Autodesk Inventor part; units mm, degrees
ref_plane "YZ Plane" through (0, 0, 0) normal (1, 0, 0) x (0, 1, 0)
ref_plane "XZ Plane" through (0, 0, 0) normal (0, 1, 0) x (-1, 0, 0)
ref_plane "XY Plane" through (0, 0, 0) normal (0, 0, 1) x (1, 0, 0)
sketch "Sketch1" plane through (0, 0, 0) normal (1, 0, 0) x (0, 1, 0)
  line L0 (40, 0) -> (40, 3)
  line L1 (40, 3) -> (10, 3)
  line L2 (10, 3) -> (10, 6)
  arc A0 (10, 6) -> (2.1459, 3) centre (5.5, 6) ccw
  line L3 (0, 0) -> (0, 3)
  line L4 (0, 3) -> (2.1459, 3)
  line L5 (40, 0) -> (0, 0)
  circle A1 centre (5.5, 6) radius 1.5
  dimension "d7" = 3
extrude "Extrusion1" add sketch "Sketch1" along normal blind 20
sketch "Sketch2" plane through (0, 0, 0) normal (0, -1, 0) x (1, 0, 0)
  line L0 (0, 0) -> (20, 0)
  line L1 (18.5, 0) -> (16.5, 0)
  line L2 (15, 1.5) -> (15, 1.5)
  line L3 (0, 3) -> (20, 3)
  line L4 (16.5, 3) -> (18.5, 3)
  line L5 (20, 1.5) -> (20, 1.5)
  arc A0 (20, 1.5) -> (18.5, 3) centre (18.5, 1.5) ccw
  arc A1 (18.5, 0) -> (20, 1.5) centre (18.5, 1.5) ccw
  arc A2 (16.5, 3) -> (15, 1.5) centre (16.5, 1.5) ccw
  arc A3 (15, 1.5) -> (16.5, 0) centre (16.5, 1.5) ccw
  line L6 (0, 6) -> (0, 3)
  line L7 (1.5, 3) -> (3.5, 3)
  line L8 (5, 1.5) -> (5, 1.5)
  line L9 (3.5, 0) -> (1.5, 0)
  line L10 (0, 0) -> (0, 3)
  line L11 (0, 1.5) -> (0, 1.5)
  arc A4 (5, 1.5) -> (3.5, 3) centre (3.5, 1.5) ccw
  arc A5 (3.5, 0) -> (5, 1.5) centre (3.5, 1.5) ccw
  arc A6 (1.5, 3) -> (0, 1.5) centre (1.5, 1.5) ccw
  arc A7 (0, 1.5) -> (1.5, 0) centre (1.5, 1.5) ccw
  point P0 (15, 0)
  point P1 (15, 3)
  point P2 (5, 3)
  point P3 (5, 0)
  dimension "d10" = 5
  dimension "d11" = 3
  dimension "d12" = 5
  dimension "d13" = 3
  dimension "d14" = 1.5
  dimension "d15" = 5
  dimension "d16" = 3
  dimension "d17" = 5
  dimension "d18" = 3
  dimension "d19" = 1.5
extrude "Extrusion2" add sketch "Sketch2" along normal blind 19 contours A7 A6 L3 A4 A5 L0 | A3 A2 L3 A0 A1 L0
ref_plane "Work Plane1" through (18.5, -19, 3) normal (0, -1, 0) x (1, 0, 0)
sketch "Sketch4" plane through (20, 0, 0) normal (1, 0, 0) x (0, 0, -1)
  line L0 (-3, -19) -> (0, -19)
  line L1 (0, -19) -> (0, -29)
  line L2 (0, -29) -> (-6, -29)
  arc A0 (-3, -21.1459) -> (-6, -29) centre (-6, -24.5) ccw
  line L3 (-3, -19) -> (-3, -21.1459)
  circle A1 centre (-6, -24.5) radius 1.5
  point P0 (0, 0)
  dimension "d31" = 3
extrude "Extrusion3" add sketch "Sketch4" against normal blind 20
sketch "Sketch5" plane through (0, 40, 3) normal (0, 1, 0) x (1, 0, 0)
  line L0 (0, 3) -> (20, 3)
  line L1 (20, 3) -> (20, 15)
  line L2 (20, 15) -> (0, 15)
  line L3 (0, 0) -> (0, 3)
  line L4 (0, 15) -> (0, 3)
  line L5 (0, 3) -> (20, 3)
  circle A0 centre (17, 10) radius 1.5
  circle A1 centre (3, 10) radius 1.5
  dimension "d34" = 12
  dimension "d35" = 20
  dimension "d36" = 12
  dimension "d37" = 20
  dimension "d40" = 3
  dimension "d43" = 3
extrude "Extrusion4" add sketch "Sketch5" against normal blind 5
sketch "Sketch6" plane through (20, -29, 0) normal (0, -1, 0) x (1, 0, 0)
  line L0 (-20, 0) -> (-20, -12)
  line L1 (-20, 0) -> (-20, -12)
  line L2 (-20, -12) -> (0, -12)
  line L3 (-1.5, 0) -> (0, 0)
  line L4 (0, -12) -> (0, 0)
  line L5 (0, 0) -> (-20, 0)
  line L6 (-16.5, 0) -> (-3.5, 0)
  circle A0 centre (-17, -7) radius 1.5
  circle A1 centre (-17, -7) radius 1.5
  circle A2 centre (-3, -7) radius 1.5
  circle A3 centre (-3, -7) radius 1.5
  dimension "d46" = 12
  dimension "d47" = 20
  dimension "d48" = 12
  dimension "d49" = 20
  dimension "d50" = 3
  dimension "d51" = 3
extrude "Extrusion5" add sketch "Sketch6" against normal blind 5
Verification items for the finished model (mm, model axes). A direction names the side the tool comes from. Coordinates: 2 decimals unless noted, no trailing zeros. Order: outer loops, then holes, each group sorted by start corner. A loop starts at its lowest first (then second) coordinate and runs counter-clockwise, first axis right, second up. Notation, with made-up numbers: (71.5, 36) -> (100.5, 36) arc R19 ccw to (100.5, 56) -> close; hole circle Ø9 at (65.25, 37). An arc over 180 degrees is marked (long way). Put each result on its own line as item: value. Start each with the question number.
1) Go/stop test with flat-tipped pins: pin 1 (10 mm diameter, centred on y = -13, z = 3, fed in from -X); pin 2 (2.5 mm diameter, centred on x = 17, z = -7, fed in from +Y); pin 3 (1.5 mm diameter, centred on x = 8, z = 5, fed in from +Y); pin 4 (6 mm diameter, centred on x = 7, y = 24.5, fed in from +Z). Record where each tip stops, or that it passes through.
2) Cross-section at C-C (y = 17). Enter the section's corners in (x, z).
3) Material ranges on L1, parallel to X at y = 38.35, z = -7; L2, parallel to Y at x = 12, z = -3.75; L3, parallel to Y at x = 15, z = 2.5, recorded low to high.
4) Cross-section at B-B (z = -7). Enter the section's corners in (x, y).
5) Tool access check on faces 4 (the cylindrical face through (15, -9.4, 1.5)), 5 (the flat face through (0.3, 0, 2.64)), 6 (the flat face through (10, 35, -6)), 7 (the cylindrical face through (9.9, 4.3, 6.9)), 8 (the flat face through (19.64, 0, 0.3)). Record the directions out of +Z, -Z, +X, -X, +Y, -Y that give a thin tool (end or side, any length) a straight path to the whole face; none if there is none.
6) Release check for a two-part mould opening along Y. For faces 1 (the flat face through (0, -25, -1)), 2 (the flat face through (19.64, -19, 2.7)), 3 (the flat face through (10, 10, 4)) record: pulls with the +Y half, pulls with the -Y half, needs draft (parallel to the pull), parting line crosses it, or undercut.
7) Cross-section at A-A (x = 14). Enter the section's corners in (y, z), plus the area to 3 significant figures.
Geometry check:
1. pin 1: stops at x = 0
1. pin 2: passes through
1. pin 3: stops at y = 10
1. pin 4: stops at z = 3
2. outline: (0, 0) -> (20, 0) -> (20, 3) -> (0, 3) -> close
3. L1: x = 0 to 1.5, 4.5 to 15.5, 18.5 to 20
3. L2: y = -29 to -24, 35 to 40
3. L3: y = -29 to -19, 0 to 40
4. outline: (0, -29) -> (1.5, -29) -> (1.5, -24) -> (0, -24) -> close; (0, 35) -> (1.5, 35) -> (1.5, 40) -> (0, 40) -> close; (4.5, -29) -> (15.5, -29) -> (15.5, -24) -> (4.5, -24) -> close; (4.5, 35) -> (15.5, 35) -> (15.5, 40) -> (4.5, 40) -> close; (18.5, -29) -> (20, -29) -> (20, -24) -> (18.5, -24) -> close; (18.5, 35) -> (20, 35) -> (20, 40) -> (18.5, 40) -> close
5. face 4: none
5. face 5: +Z, -X
5. face 6: -Z, +X, -X
5. face 7: +X, -X
5. face 8: -Z, +X
6. face 1: needs draft
6. face 2: undercut
6. face 3: pulls with the +Y half
7. outline: (-29, -12) -> (-24, -12) -> (-24, 0) -> (-19, 0) -> (-19, 3) -> (-21.15, 3) arc R4.5 ccw (long way) to (-29, 6) -> close; (0, 0) -> (35, 0) -> (35, -12) -> (40, -12) -> (40, 3) -> (10, 3) -> (10, 6) arc R4.5 ccw (long way) to (2.15, 3) -> (0, 3) -> close; hole circle Ø3 at (-24.5, 6); hole circle Ø3 at (5.5, 6)
7. area: 371 mm^2
